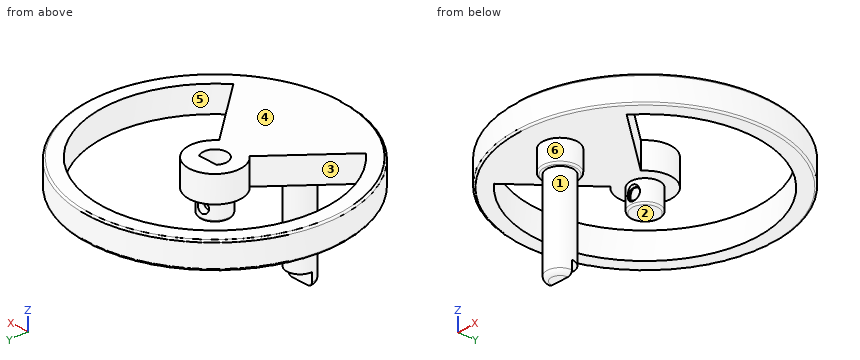
from build123d import *

# Parameters (mm, degrees)
ESQUISSE2_R             = 14.79822015
BOSS_EXTRU_1_DEPTH      = 3
CONG_2_R                = 0.2
CONG_3_R                = 0.2
ESQUISSE3_R             = 1.5
BOSS_EXTRU_2_DEPTH      = 13
CONG_4_R                = 0.5
ENL_V_MAT_EXTRU_1_DEPTH = 3.5
ESQUISSE5_R             = 1.675
BOSS_EXTRU_3_DEPTH      = 2.5
ENL_V_START             = -5
ENL_V_MAT_EXTRU_2_DEPTH = 5
CONG_6_R                = 0.2
ESQUISSE8_R             = 2
ESQUISSE8_R_2           = 1.5
BOSS_EXTRU_4_DEPTH      = 2.5
CONG_7_R                = 0.2
ENL_V_MAT_EXTRU_3_REACH = 27.888
ESQUISSE14_W            = 6.151008923
ESQUISSE14_H            = 1.920006843
ENL_V_MAT_EXTRU_4_DEPTH = 1.5


with BuildPart() as part:
    # Esquisse2 → Boss.-Extru.1 (new body)
    with BuildSketch(Plane(origin=(0, 0, 2), x_dir=(-1, 0, 0), z_dir=(0, 0, -1))):
        with Locations((0, -2)):
            Circle(ESQUISSE2_R)
    extrude(amount=BOSS_EXTRU_1_DEPTH)

    # Congé2
    cong_2_edges = [part.edges().sort_by_distance(p)[0] for p in [
        (14.79822015, -2, -1),
    ]]
    fillet(cong_2_edges, radius=CONG_2_R)

    # Congé3
    cong_3_edges = [part.edges().sort_by_distance(p)[0] for p in [
        (14.79822015, -2, 2),
    ]]
    fillet(cong_3_edges, radius=CONG_3_R)

    # Esquisse3 → Boss.-Extru.2 (add)
    with BuildSketch(Plane(origin=(0, 0, -1), x_dir=(-1, 0, 0), z_dir=(0, 0, -1))):
        with Locations(Location((0, -12, 0), (0, 0, 180))):
            Circle(ESQUISSE3_R)
    extrude(amount=BOSS_EXTRU_2_DEPTH)

    # Congé4
    cong_4_edges = [part.edges().sort_by_distance(p)[0] for p in [
        (-1.5, -12, -14),
    ]]
    fillet(cong_4_edges, radius=CONG_4_R)

    # Esquisse4 → Enlèv. mat.-Extru.1 (cut)
    with BuildSketch(Plane(origin=(0, 0, -1), x_dir=(-1, 0, 0), z_dir=(0, 0, -1))):
        with BuildLine():
            Line((-1.1, -1.175), (1.1, -1.175))
            ThreePointArc((1.1, -1.175), (0, -3.375), (-1.1, -1.175))
        make_face()
    extrude(amount=-ENL_V_MAT_EXTRU_1_DEPTH, mode=Mode.SUBTRACT)

    # Esquisse5 → Boss.-Extru.3 (add)
    with BuildSketch(Plane(origin=(0, 0, -1), x_dir=(-1, 0, 0), z_dir=(0, 0, -1))):
        with Locations((0, -2)):
            Circle(ESQUISSE5_R)
    extrude(amount=BOSS_EXTRU_3_DEPTH)

    # Esquisse6 → Enlèv. mat.-Extru.2 (cut)
    with BuildSketch(Plane.XY.offset(2).offset(ENL_V_START)):
        with BuildLine():
            Line((1.1, -1.175), (-1.1, -1.175))
            ThreePointArc((-1.1, -1.175), (0, -3.375), (1.1, -1.175))
        make_face()
    extrude(amount=ENL_V_MAT_EXTRU_2_DEPTH, mode=Mode.SUBTRACT)

    # Congé6
    cong_6_edges = [part.edges().sort_by_distance(p)[0] for p in [
        (1.675, -2, -3.5),
    ]]
    fillet(cong_6_edges, radius=CONG_6_R)

    # Esquisse8 → Boss.-Extru.4 (add)
    with BuildSketch(Plane(origin=(0, 0, -1), x_dir=(-1, 0, 0), z_dir=(0, 0, -1))):
        with Locations((0, -12)):
            Circle(ESQUISSE8_R)
        with Locations(Location((0, -12, 0), (0, 0, 180))):
            Circle(ESQUISSE8_R_2, mode=Mode.SUBTRACT)
    extrude(amount=BOSS_EXTRU_4_DEPTH)

    # Congé7
    cong_7_edges = [part.edges().sort_by_distance(p)[0] for p in [
        (2, -12, -3.5),
    ]]
    fillet(cong_7_edges, radius=CONG_7_R)

    # Esquisse9 → Trou taraudé M1.61 (revolve, cut)
    with BuildSketch(Plane(origin=(0.228696217, -3.659314027, -2.244412235), x_dir=(0.9906352400032369, 0.1365350550727882, 0), z_dir=(0, 0, 1))):
        Polygon((0, 0), (0, 18.355114173), (0.625, 18.355114173), (0.625, 0.2), (0.825, 0), align=None)
    revolve(axis=Axis((1.095693817, -9.949847801, -2.244412235), (-0.13653505507278818, 0.9906352400032369, 0)), mode=Mode.SUBTRACT)

    # Esquisse11 → Enlèv. mat.-Extru.3 (cut, up to next)
    with BuildSketch(Plane(origin=(0, 0, -1), x_dir=(-1, 0, 0), z_dir=(0, 0, -1)), mode=Mode.PRIVATE) as enl_v_mat_extru_3_sk1:
        with BuildLine():
            Line((-1.928362829, -4.298133329), (-8.356238926, -11.958577761))
            ThreePointArc((-8.356238926, -11.958577761), (0, 11), (8.356238926, -11.958577761))
            Line((8.356238926, -11.958577761), (1.928362829, -4.298133329))
            ThreePointArc((1.928362829, -4.298133329), (0, 1), (-1.928362829, -4.298133329))
        make_face()
    enl_v_mat_extru_3_tool1 = extrude(enl_v_mat_extru_3_sk1.sketch, amount=-ENL_V_MAT_EXTRU_3_REACH, mode=Mode.PRIVATE) & part.part
    add(enl_v_mat_extru_3_tool1.solids().sort_by_distance((-5.408009, -7.9054, -1))[0], mode=Mode.SUBTRACT)

    # Esquisse14 → Enlèv. mat.-Extru.4 (cut)
    with BuildSketch(Plane(origin=(0, 0, -14), x_dir=(-1, 0, 0), z_dir=(0, 0, -1))):
        with Locations((-0.122541976, -11.039996579)):
            Rectangle(ESQUISSE14_W, ESQUISSE14_H)
    extrude(amount=-ENL_V_MAT_EXTRU_4_DEPTH, mode=Mode.SUBTRACT)


solid = part.part
Here's how the part is built. I have some questions about the finished solid (model axes, mm). Face numbers are marked on the shaded views. A direction names the side the tool comes from. Coordinates: 2 decimals unless noted, no trailing zeros. Loops run counter-clockwise (first coordinate to the right, second up) from the corner with the lowest first, then second, coordinate; pieces in that order, holes last. Notation, with made-up numbers: (19.5, 1.25) -> (71.5, 1.25) arc R18 ccw to (71.5, 30.25) -> close; hole circle Ø7 at (84, 72). An arc over 180 degrees is marked (long way). Use one line per item in the form item = value. Start each with the question number.
(1) If we section it at B-B (x = 0): Give the number of separate pieces and of enclosed holes in the cut face, then the cut area to 3 significant figures.
(2) If we section it at A-A (y = -2): Please give me the cut outline in (x, z) (3 decimals).
(3) Will these pins go through, and if not, where does the flat tip stop? pin 1 (4 mm diameter, centred on x = 4.5, z = -0.5, fed in from -Y); pin 2 (1.8 mm diameter, centred on x = 1, y = -11, fed in from -Z); pin 3 (1.7 mm diameter, centred on x = 0, z = -13, fed in from +Y).
(4) Please list where these lines run through material, in increasing order: line 1 along Y through (x, z) = (0, 0.55) (3 decimals); line 2 along Y through (x, z) = (0, -1.05) (3 decimals); line 3 along X through (y, z) = (-1.75, -0.5).
(5) We'd pull the mould along X, two halves only. Please class the marked faces 4, 5 and 6: pulls with the +X half, pulls with the -X half, needs draft (parallel to the pull), parting line crosses it, or undercut.
(6) On a 3-axis mill with a long thin cutter (end or side, diameter ignored), from which of +Z, -Z, +X, -X, +Y, -Y can I reach the whole of each face in a straight line? I mean the marked faces 1, 2 and 3. Say none if no direction works.
Verdict:
q1.separate_pieces = 4
q1.enclosed_holes = 0
q1.area = 93.9 mm²
q2.outline = (-14.798, -0.8) arc R0.2 ccw to (-14.598, -1) -> (-13, -1) -> (-13, 2) -> (-14.598, 2) arc R0.2 ccw to (-14.798, 1.8) -> close; (-3, -1) -> (-1.675, -1) -> (-1.675, -3.3) arc R0.2 ccw to (-1.475, -3.5) -> (1.475, -3.5) arc R0.2 ccw to (1.675, -3.3) -> (1.675, -1) -> (3, -1) -> (3, 2) -> (1.375, 2) -> (1.375, -3) -> (-1.375, -3) -> (-1.375, 2) -> (-3, 2) -> close; (13, -1) -> (14.598, -1) arc R0.2 ccw to (14.798, -0.8) -> (14.798, 1.8) arc R0.2 ccw to (14.598, 2) -> (13, 2) -> close
q3.pin_1 = -16.59
q3.pin_2 = -12.5
q3.pin_3 = -10.5
q4.line_1 = -16.798 to -3.375, -1.175 to 1, 11 to 12.798
q4.line_2 = -14 to -10, -3.675 to -3.375, -1.175 to -0.325
q4.line_3 = -14.8 to -13, -2.99 to -1.35, 1.35 to 2.99, 13 to 14.8
q5.face_4 = needs draft
q5.face_5 = undercut
q5.face_6 = parting line crosses it
q6.face_1 = -Z
q6.face_2 = -Z, +X, -X, +Y
q6.face_3 = +Z, -Z
